Part model, mm, in its own coordinate system. A direction names the side the tool comes from. Coordinates: 2 decimals unless noted, no trailing zeros. Order: outer loops, then holes, each group sorted by start corner. A loop starts at its lowest first (then second) coordinate and runs counter-clockwise, first axis right, second up. Notation, with made-up numbers: M 56.5,89 L 101.5,89 A13 ccw 101.5,107 Z; hole C -10.75,-28.5 d8. An arc over 180 degrees is marked long. Answer in a Markdown table with one row per item. Add a question column.
from build123d import *

# Parameters (mm, degrees)
F0_W           = 40
F0_H           = 80
F1_DEPTH       = 30
F1_TAPER       = 1
F3_D           = 9
F3_CBORE_D     = 15
F3_CBORE_DEPTH = 10


with BuildPart() as f1:
    # F0 (on Top) → F1 (new body, symmetric)
    with BuildSketch(Plane.XY):
        with Locations((0, -2.7505960315)):
            Rectangle(F0_W, F0_H)
    extrude(amount=F1_DEPTH, both=True, taper=F1_TAPER)

    # F3 (through all)
    with Locations(Plane.XY.offset(30)):
        with Locations((-5, -12.7505960315)):
            CounterBoreHole(F3_D / 2, F3_CBORE_D / 2, F3_CBORE_DEPTH)


solid = f1.part
(1) 3-axis set-ups, long thin cutter, end or side, ignore diameter. For faces 3 (the cylindrical face through (-10.952, -17.314, 25.07)), 4 (the cylindrical face through (-4.024, -17.144, -5.35)): which of +Z, -Z, +X, -X, +Y, -Y reach the whole face in a straight line?
(2) Slice it at A-A (z = 13). List the corners of the cut face in (x, y), and give its area (3 significant figures).
(3) Wall check: line 1 (Y direction, x = -5, z = 26); line 2 (X direction, y = -10.5, z = -12); line 3 (Y direction, x = -5, z = -3). Give the ranges that are in metal, low to high.
(4) Drop flat-ended pins along their axis: P1, Ø4, axis at x = -13.5, z = 17.5, coming from the +Y side; P2, Ø1.5, axis at x = -10.5, z = -10, coming from the +Y side; P3, Ø3, axis at x = -12.5, z = 2.5, coming from the +Y side. Give the stop position or say it passes through.
(5) Pull direction Y, two halves, no side cores. Call faces 1 (the flat face through (0, -2, 30)), 2 (the flat face through (-5, -18, 20)): pulls with the +Y half, pulls with the -Y half, needs draft (parallel to the pull), parting line crosses it, or undercut.
Computed:
| question | item | result |
|---|---|---|
| 1 | face 3 | +Z |
| 1 | face 4 | +Z, -Z |
| 2 | outline | M -19.77,-42.52 L 19.77,-42.52 L 19.77,37.02 L -19.77,37.02 Z; hole C -5,-12.75 d9 |
| 2 | area | 3,080 mm^2 |
| 3 | line 1 | y = -42.3 to -20.25, -5.25 to 36.8 |
| 3 | line 2 | x = -19.79 to -8.9, -1.1 to 19.79 |
| 3 | line 3 | y = -42.7 to -17.25, -8.25 to 37.2 |
| 4 | P1 | stops at y = 36.98 |
| 4 | P2 | stops at y = 37.09 |
| 4 | P3 | stops at y = 37.23 |
| 5 | face 1 | needs draft |
| 5 | face 2 | undercut |
